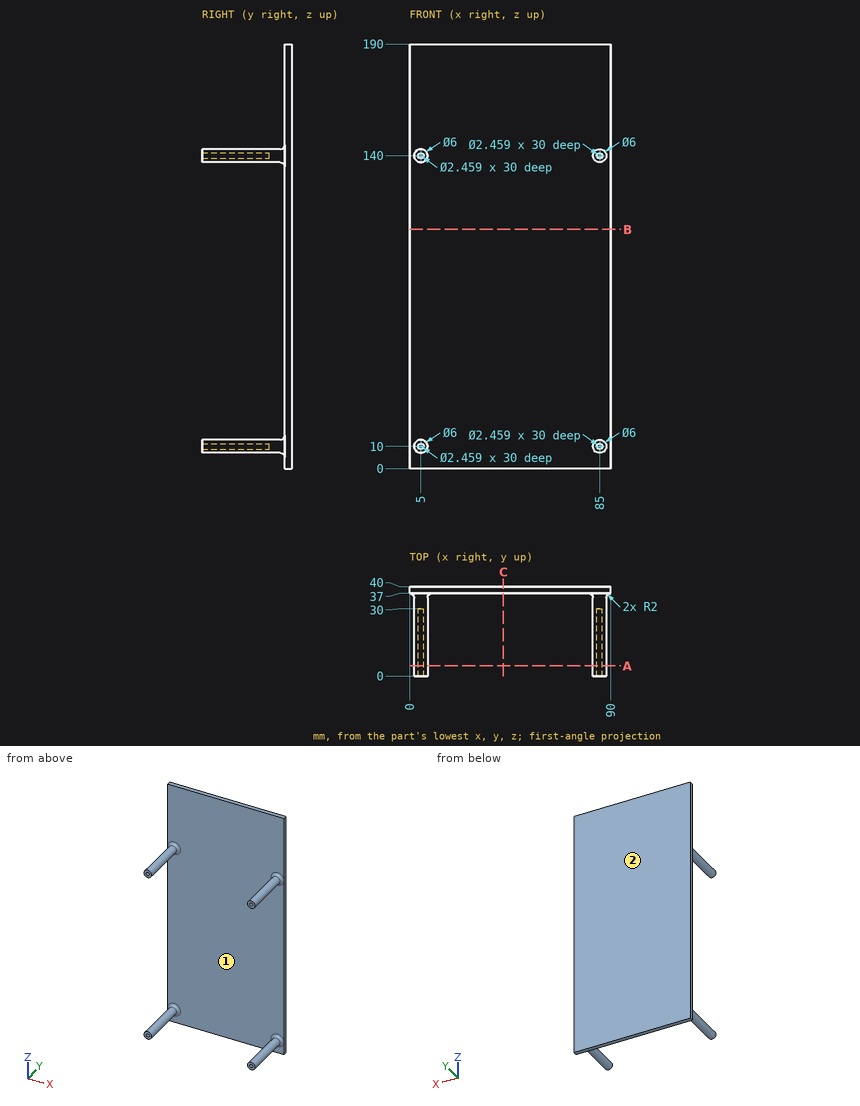
Part print with two shaded views. Sizes in mm from the minimum x, y, z corner. A direction names the side the tool comes from. Round coordinates to 2 decimals unless told otherwise and drop trailing zeros. Loops run counter-clockwise (first coordinate to the right, second up) from the corner with the lowest first, then second, coordinate; pieces in that order, holes last. Notation, with made-up numbers: M -14.75,-8.75 L 35.25,-8.75 A22 ccw 35.25,0.25 Z; hole C -32,15 d4. An arc over 180 degrees is marked long. Return JSON: item names as keys, results as strings. Group by question number.
(1) Saw through at A-A, the plane y = 4.5. List the corners of the cut face in (x, z).
(2) Drop flat-ended pins along their axis: P1, Ø1.2, axis at x = 85, z = 9.5, coming from the -Y side; P2, Ø6, axis at y = 9, z = 137.5, coming from the -X side. Give the stop position or say it passes through.
(3) Saw through at B-B, the plane z = 107. List the corners of the cut face in (x, y).
(4) Wall check: probe 1 along Z at (x, y) = (85, 21.5); probe 2 along X at (y, z) = (15.75, 140); probe 3 along X at (y, z) = (17, 139) (1 decimal). Give the ranges that are in metal, low to high. Write a range as [from, to].
(5) Saw through at C-C, the plane x = 42. List the corners of the cut face in (y, z).
(6) Tool access for the marked faces 1 and 2: list every direction of +Z, -Z, +X, -X, +Y, -Y with a clear straight run to the whole face (end or side of a thin tool).
Answer list:
{
 "1": {"outline": "C 5,10 d6; C 5,140 d6; C 85,10 d6; C 85,140 d6; hole C 5,10 d2.46; hole C 5,140 d2.46; hole C 85,10 d2.46; hole C 85,140 d2.46"},
 "2": {"P1": "y = 30", "P2": "x = 2"},
 "3": {"outline": "M 0,37 L 90,37 L 90,40 L 0,40 Z"},
 "4": {"probe 1": "[7, 8.77], [11.23, 13], [137, 138.77], [141.23, 143]", "probe 2": "[2, 3.77], [6.23, 8], [82, 83.77], [86.23, 88]", "probe 3": "[2.2, 4.3], [5.7, 7.8], [82.2, 84.3], [85.7, 87.8]"},
 "5": {"outline": "M 37,0 L 40,0 L 40,190 L 37,190 Z"},
 "6": {"face 1": "-Y", "face 2": "+Z, -Z, +X, -X, +Y"}
}
